Work out the finished part from the listing and answer in its coordinate system (mm). A direction names the side the tool comes from. Coordinates: 2 decimals unless noted, no trailing zeros. Order: outer loops, then holes, each group sorted by start corner. A loop starts at its lowest first (then second) coordinate and runs counter-clockwise, first axis right, second up. Notation, with made-up numbers: (69.5, 50.25) -> (124.5, 50.25) arc R29 cw to (124.5, 73.25) -> close; hole circle Ø9 at (3, -8). An arc over 180 degrees is marked (long way). Write item = value, one per line. Start each with the question number.
Q1. The part is cut by section B-B, the plane y = 17.5. Determine the outline of the cut face in (x, z), plus the area to 3 significant figures.
Q2. Which of the six approach directions +Z, -Z, +X, -X, +Y, -Y give full straight-line access (tool end or side, diameter ignored) to faces 5 (the flat face through (7, 41, -17.5)), 6 (the flat face through (7, 41, -32.5)), 7 (the flat face through (0, 41, -25))?
Q3. The part is cut by section C-C, the plane z = -24. Determine the outline of the cut face in (x, y), plus the area to 3 significant figures.
Q4. Flat-ended cylindrical pins translate along their axes: pin 1 (6 mm diameter, centred on y = 39.5, z = -24, fed in from +X); pin 2 (6 mm diameter, centred on x = 8.5, y = 42, fed in from +Z); pin 3 (6 mm diameter, centred on x = 63, y = 16.5, fed in from +Z); pin 4 (3.5 mm diameter, centred on x = 7.5, y = 42, fed in from -Z). Find the tip coordinate at first contact, or state that the pin passes through.
Q5. Straight lines are drawn through the part: L1, parallel to Y at x = 125, z = -20.5; L2, parallel to X at y = 18, z = -4.5; L3, parallel to X at y = 21, z = -3. For each, find the intervals that lie inside material, in ascending order. Write a range as from..to.
Q6. For a pull along Y with two mould halves and no side action, classify faces 1 (the cylindrical face through (137, 21, -25)), 2 (the flat face through (15, 41, -25)), 3 (the flat face through (7, 47, -25)), 4 (the cylindrical face through (-113, 21, -25)) as +Y half, -Y half, draft (parallel to the pull), parting line (faces both ways), or undercut.
Q7. The part is cut by section D-D, the plane x = -60. Determine the outline of the cut face in (y, z), plus the area to 3 significant figures.
Q8. The part is cut by section A-A, the plane x = 125. Determine the outline of the cut face in (y, z), plus the area to 3 significant figures.
```python
from build123d import *

# Parameters (mm, degrees)
SKETCH1_W           = 300
SKETCH1_H           = 50
BOSS_EXTRUDE1_DEPTH = 35
SKETCH2_W           = 15
SKETCH2_H           = 15
BOSS_EXTRUDE2_DEPTH = 12
CUT_EXTRUDE1_REACH  = 166.952
SKETCH3_R           = 12.5


with BuildPart() as part:
    # Sketch1 → Boss-Extrude1 (new body)
    with BuildSketch(Plane(origin=(0, 0, 0), x_dir=(1, 0, 0), z_dir=(0, 1, 0))):
        with Locations((0, 25)):
            Rectangle(SKETCH1_W, SKETCH1_H)
    extrude(amount=BOSS_EXTRUDE1_DEPTH)

    # Sketch2 → Boss-Extrude2 (add)
    with BuildSketch(Plane(origin=(0, 35, 0), x_dir=(1, 0, 0), z_dir=(0, 1, 0))):
        with Locations((7.5, 25)):
            Rectangle(SKETCH2_W, SKETCH2_H)
    extrude(amount=BOSS_EXTRUDE2_DEPTH)

    # Sketch3 → Cut-Extrude1 (cut, up to next)
    with BuildSketch(Plane.XY, mode=Mode.PRIVATE) as cut_extrude1_sk1:
        with Locations((-125, 17.5)):
            Circle(SKETCH3_R)
    cut_extrude1_tool1 = extrude(cut_extrude1_sk1.sketch, amount=-CUT_EXTRUDE1_REACH, mode=Mode.PRIVATE) & part.part
    # Sketch3 → Cut-Extrude1 (cut, up to next)
    with BuildSketch(Plane.XY, mode=Mode.PRIVATE) as cut_extrude1_sk2:
        with Locations((125, 17.5)):
            Circle(SKETCH3_R)
    cut_extrude1_tool2 = extrude(cut_extrude1_sk2.sketch, amount=-CUT_EXTRUDE1_REACH, mode=Mode.PRIVATE) & part.part
    add(cut_extrude1_tool1.solids().sort_by_distance((-125, 17.5, 0))[0], mode=Mode.SUBTRACT)
    add(cut_extrude1_tool2.solids().sort_by_distance((125, 17.5, 0))[0], mode=Mode.SUBTRACT)


solid = part.part
```
Model answer:
q1.outline = (-150, -50) -> (-137.5, -50) -> (-137.5, 0) -> (-150, 0) -> close; (-112.5, -50) -> (112.5, -50) -> (112.5, 0) -> (-112.5, 0) -> close; (137.5, -50) -> (150, -50) -> (150, 0) -> (137.5, 0) -> close
q1.area = 12,500 mm2
q2.face_5 = +Z, +X, -X, +Y
q2.face_6 = -Z, +X, -X, +Y
q2.face_7 = +Z, -Z, -X, +Y
q3.outline = (-150, 0) -> (150, 0) -> (150, 35) -> (15, 35) -> (15, 47) -> (0, 47) -> (0, 35) -> (-150, 35) -> close; hole circle Ø25 at (-125, 17.5); hole circle Ø25 at (125, 17.5)
q3.area = 9,700 mm2
q4.pin_1 = 15
q4.pin_2 = -17.5
q4.pin_3 = 0
q4.pin_4 = -32.5
q5.L1 = 0..5, 30..35
q5.L2 = -150..-137.49, -112.51..112.51, 137.49..150
q5.L3 = -150..-137, -113..113, 137..150
q6.face_1 = undercut
q6.face_2 = draft
q6.face_3 = +Y half
q6.face_4 = undercut
q7.outline = (0, -50) -> (35, -50) -> (35, 0) -> (0, 0) -> close
q7.area = 1,750 mm2
q8.outline = (0, -50) -> (5, -50) -> (5, 0) -> (0, 0) -> close; (30, -50) -> (35, -50) -> (35, 0) -> (30, 0) -> close
q8.area = 500 mm2
